The listing builds one solid part. Answer for the finished solid, in the listing's coordinates (mm). A direction names the side the tool comes from. Give positions to 0.01 mm unless a question says otherwise; leave off trailing zeros. Return JSON: item names as keys, results as strings.
from build123d import *

# Parameters (mm, degrees)
CYLINDER014005872_R                            = 40.05
CYLINDER014005872_DEPTH                        = 16
CYLINDER014005874_R                            = 3.65
CYLINDER014005874_DEPTH                        = 4
CYLINDER014005873_R                            = 2.15
CYLINDER014005873_DEPTH                        = 24
FUSION001089102007007003001_PLACEMENT_ANGLE    = 60
FUSION001089102007007003002_PLACEMENT_ANGLE    = 120
FUSION001089102007007003003_PLACEMENT_ANGLE    = 180
FUSION001089102007007003004_PLACEMENT_ANGLE    = 240
FUSION001089102007007003005_PLACEMENT_ANGLE    = 60
BOX002_W                                       = 7
BOX002_H                                       = 10
BOX002_DEPTH                                   = 3.4
PRISM003_DEPTH                                 = 3.4
CYLINDER014005875_R                            = 2.15
CYLINDER014005875_DEPTH                        = 16
FUSION001089102007007003008001_PLACEMENT_ANGLE = 60
FUSION001089102007007003008002_PLACEMENT_ANGLE = 120
FUSION001089102007007003008003_PLACEMENT_ANGLE = 180
FUSION001089102007007003008004_PLACEMENT_ANGLE = 240
FUSION001089102007007003008005_PLACEMENT_ANGLE = 60
BOX003_W                                       = 4.1
BOX003_H                                       = 8
BOX003_DEPTH                                   = 10
CYLINDER014005876_R                            = 2.65
CYLINDER014005876_DEPTH                        = 14
PRISM004_DEPTH                                 = 4.2
BOX004_W                                       = 4.1
BOX004_H                                       = 8
BOX004_DEPTH                                   = 10
CYLINDER014005877_R                            = 2.65
CYLINDER014005877_DEPTH                        = 14
PRISM005_DEPTH                                 = 4.2
CYLINDER014005871_R                            = 36
CYLINDER014005871_DEPTH                        = 16
BOX_W                                          = 10
BOX_H                                          = 44
BOX_DEPTH                                      = 16
CYLINDER014005870_R                            = 53
CYLINDER014005870_DEPTH                        = 16
CHAMFER012_SIZE                                = 0.75


with BuildPart() as obj1:
    # Cylinder014005872 → Cylinder014005872 (new body)
    with BuildSketch(Plane.XY.offset(0.1)):
        Circle(CYLINDER014005872_R)
    extrude(amount=CYLINDER014005872_DEPTH)


with BuildPart() as obj2:
    # Cylinder014005874 → Cylinder014005874 (new body)
    with BuildSketch(Plane(origin=(45, 0, 4), x_dir=(1, 0, 0), z_dir=(0, 0, 1))):
        Circle(CYLINDER014005874_R)
    extrude(amount=CYLINDER014005874_DEPTH)


with BuildPart() as obj3:
    # Cylinder014005873 → Cylinder014005873 (new body)
    with BuildSketch(Plane(origin=(45, 0, -16), x_dir=(1, 0, 0), z_dir=(0, 0, 1))):
        Circle(CYLINDER014005873_R)
    extrude(amount=CYLINDER014005873_DEPTH)

    # Fusion001089102007007003: union obj2
    add(obj2.part)


with BuildPart() as obj4:
    # Fusion001089102007007003001 base: copy of obj3
    add(obj3.part)


with BuildPart() as obj4_1:
    # Fusion001089102007007003001 placement: moved
    add(obj4.part.rotate(Axis((0, 0, 0), (0, 0, 1)), FUSION001089102007007003001_PLACEMENT_ANGLE))


with BuildPart() as obj5:
    # Fusion001089102007007003002 base: copy of obj3
    add(obj3.part)


with BuildPart() as obj5_1:
    # Fusion001089102007007003002 placement: moved
    add(obj5.part.rotate(Axis((0, 0, 0), (0, 0, 1)), FUSION001089102007007003002_PLACEMENT_ANGLE))


with BuildPart() as obj6:
    # Fusion001089102007007003003 base: copy of obj3
    add(obj3.part)


with BuildPart() as obj6_1:
    # Fusion001089102007007003003 placement: moved
    add(obj6.part.rotate(Axis((0, 0, 0), (0, 0, 1)), FUSION001089102007007003003_PLACEMENT_ANGLE))


with BuildPart() as obj7:
    # Fusion001089102007007003004 base: copy of obj3
    add(obj3.part)


with BuildPart() as obj7_1:
    # Fusion001089102007007003004 placement: moved
    add(obj7.part.rotate(Axis((0, 0, 0), (0, 0, 1)), FUSION001089102007007003004_PLACEMENT_ANGLE))


with BuildPart() as obj8:
    # Fusion001089102007007003005 base: copy of obj3
    add(obj3.part)


with BuildPart() as obj8_1:
    # Fusion001089102007007003005 placement: moved
    add(obj8.part.rotate(Axis((0, 0, 0), (0, 0, -1)), FUSION001089102007007003005_PLACEMENT_ANGLE))


with BuildPart() as fusion001089102007007003006:
    # Fusion001089102007007003006 base: copy of obj3
    add(obj3.part)

    # Fusion001089102007007003006: union obj4, obj5, obj6, obj7, obj8
    add(obj4_1.part)
    add(obj5_1.part)
    add(obj6_1.part)
    add(obj7_1.part)
    add(obj8_1.part)


with BuildPart() as krychle002:
    # Box002 → Box002 (new body)
    with BuildSketch(Plane(origin=(-3.5, 0, 0), x_dir=(1, 0, 0), z_dir=(0, 0, 1))):
        with Locations((3.5, 5)):
            Rectangle(BOX002_W, BOX002_H)
    extrude(amount=BOX002_DEPTH)


with BuildPart() as m4x003:
    # prism003 → prism003 (new body)
    with BuildSketch(Plane(origin=(0, 0, 0), x_dir=(0, 1, 0), z_dir=(0, 0, 1))):
        Polygon((4.21, 0), (2.105, 3.645967), (-2.105, 3.645967), (-4.21, 0), (-2.105, -3.645967), (2.105, -3.645967), align=None)
    extrude(amount=PRISM003_DEPTH)


with BuildPart() as m4nut:
    # Cylinder014005875 → Cylinder014005875 (new body)
    with BuildSketch(Plane.XY.offset(-8)):
        Circle(CYLINDER014005875_R)
    extrude(amount=CYLINDER014005875_DEPTH)

    # Fusion001089102007007003008: union Krychle002, M4X003
    add(krychle002.part)
    add(m4x003.part)


with BuildPart() as m4nut_1:
    # Fusion001089102007007003008 placement: moved
    add(m4nut.part.moved(Location((0, -45, 0))))


with BuildPart() as m4nut001:
    # Fusion001089102007007003008001 base: copy of M4nut
    add(m4nut_1.part)


with BuildPart() as m4nut001_1:
    # Fusion001089102007007003008001 placement: moved
    add(m4nut001.part.rotate(Axis((0, 0, 0), (0, 0, 1)), FUSION001089102007007003008001_PLACEMENT_ANGLE))


with BuildPart() as m4nut002:
    # Fusion001089102007007003008002 base: copy of M4nut
    add(m4nut_1.part)


with BuildPart() as m4nut002_1:
    # Fusion001089102007007003008002 placement: moved
    add(m4nut002.part.rotate(Axis((0, 0, 0), (0, 0, 1)), FUSION001089102007007003008002_PLACEMENT_ANGLE))


with BuildPart() as m4nut003:
    # Fusion001089102007007003008003 base: copy of M4nut
    add(m4nut_1.part)


with BuildPart() as m4nut003_1:
    # Fusion001089102007007003008003 placement: moved
    add(m4nut003.part.rotate(Axis((0, 0, 0), (0, 0, 1)), FUSION001089102007007003008003_PLACEMENT_ANGLE))


with BuildPart() as m4nut004:
    # Fusion001089102007007003008004 base: copy of M4nut
    add(m4nut_1.part)


with BuildPart() as m4nut004_1:
    # Fusion001089102007007003008004 placement: moved
    add(m4nut004.part.rotate(Axis((0, 0, 0), (0, 0, 1)), FUSION001089102007007003008004_PLACEMENT_ANGLE))


with BuildPart() as m4nut005:
    # Fusion001089102007007003008005 base: copy of M4nut
    add(m4nut_1.part)


with BuildPart() as m4nut005_1:
    # Fusion001089102007007003008005 placement: moved
    add(m4nut005.part.rotate(Axis((0, 0, 0), (0, 0, -1)), FUSION001089102007007003008005_PLACEMENT_ANGLE))


with BuildPart() as fusion001089102007007003008006:
    # Fusion001089102007007003008006 base: copy of M4nut
    add(m4nut_1.part)

    # Fusion001089102007007003008006: union M4nut001, M4nut002, M4nut003, M4nut004, M4nut005
    add(m4nut001_1.part)
    add(m4nut002_1.part)
    add(m4nut003_1.part)
    add(m4nut004_1.part)
    add(m4nut005_1.part)


with BuildPart() as krychle003:
    # Box003 → Box003 (new body)
    with BuildSketch(Plane(origin=(0, -4, 0), x_dir=(1, 0, 0), z_dir=(0, 0, 1))):
        with Locations((2.05, 4)):
            Rectangle(BOX003_W, BOX003_H)
    extrude(amount=BOX003_DEPTH)


with BuildPart() as obj9:
    # Cylinder014005876 → Cylinder014005876 (new body)
    with BuildSketch(Plane(origin=(-4, 0, 0), x_dir=(0, 0, -1), z_dir=(1, 0, 0))):
        Circle(CYLINDER014005876_R)
    extrude(amount=CYLINDER014005876_DEPTH)


with BuildPart() as m5:
    # prism004 → prism004 (new body)
    with BuildSketch(Plane(origin=(0, 0, 0), x_dir=(0, 0, -1), z_dir=(1, 0, 0))):
        Polygon((4.6, 0), (2.3, 3.983717), (-2.3, 3.983717), (-4.6, 0), (-2.3, -3.983717), (2.3, -3.983717), align=None)
    extrude(amount=PRISM004_DEPTH)

    # Fusion001089102007007003008007: union Krychle003, obj9
    add(krychle003.part)
    add(obj9.part)


with BuildPart() as m5_1:
    # Fusion001089102007007003008007 placement: moved
    add(m5.part.moved(Location((45, 15, 0))))


with BuildPart() as krychle004:
    # Box004 → Box004 (new body)
    with BuildSketch(Plane(origin=(0, -4, 0), x_dir=(1, 0, 0), z_dir=(0, 0, 1))):
        with Locations((2.05, 4)):
            Rectangle(BOX004_W, BOX004_H)
    extrude(amount=BOX004_DEPTH)


with BuildPart() as obj10:
    # Cylinder014005877 → Cylinder014005877 (new body)
    with BuildSketch(Plane(origin=(-4, 0, 0), x_dir=(0, 0, -1), z_dir=(1, 0, 0))):
        Circle(CYLINDER014005877_R)
    extrude(amount=CYLINDER014005877_DEPTH)


with BuildPart() as m006:
    # prism005 → prism005 (new body)
    with BuildSketch(Plane(origin=(0, 0, 0), x_dir=(0, 0, -1), z_dir=(1, 0, 0))):
        Polygon((4.6, 0), (2.3, 3.983717), (-2.3, 3.983717), (-4.6, 0), (-2.3, -3.983717), (2.3, -3.983717), align=None)
    extrude(amount=PRISM005_DEPTH)

    # Fusion001089102007007003008008: union Krychle004, obj10
    add(krychle004.part)
    add(obj10.part)


with BuildPart() as m006_1:
    # Fusion001089102007007003008008 placement: moved
    add(m006.part.moved(Location((45, -15, 0))))


with BuildPart() as fusion001089102007007002:
    # Cylinder014005871 → Cylinder014005871 (new body)
    with BuildSketch(Plane.XY.offset(-8)):
        Circle(CYLINDER014005871_R)
    extrude(amount=CYLINDER014005871_DEPTH)

    # Fusion001089102007007002: union obj1, Fusion001089102007007003006, Fusion001089102007007003008006, M5, M006
    add(obj1.part)
    add(fusion001089102007007003006.part)
    add(fusion001089102007007003008006.part)
    add(m5_1.part)
    add(m006_1.part)


with BuildPart() as krychle:
    # Box → Box (new body)
    with BuildSketch(Plane(origin=(43, -22, -8), x_dir=(1, 0, 0), z_dir=(0, 0, 1))):
        with Locations((5, 22)):
            Rectangle(BOX_W, BOX_H)
    extrude(amount=BOX_DEPTH)


with BuildPart() as obj11:
    # Cylinder014005870 → Cylinder014005870 (new body)
    with BuildSketch(Plane.XY.offset(-8)):
        Circle(CYLINDER014005870_R)
    extrude(amount=CYLINDER014005870_DEPTH)

    # Fusion001089102007007003007: union Krychle
    add(krychle.part)

    # Cut009003003009003: cut Fusion001089102007007002
    add(fusion001089102007007002.part, mode=Mode.SUBTRACT)

    # Chamfer012
    chamfer012_edges = [obj11.edges().sort_by_distance(p)[0] for p in [
        (-53, 0, 8),
        (-53, 0, -8),
        (50.609127, 22, -8),
        (50.609127, 22, 8),
        (50.609127, -22, -8),
        (50.609127, -22, 8),
        (53, 0, -8),
        (-36, 0, -8),
        (-40.05, 0, 8),
        (53, 0, 8),
    ]]
    chamfer(chamfer012_edges, length=CHAMFER012_SIZE)


solid = obj11.part
Item 1: Given pin 1 Ø4 at (x, z) = (51, -1.5) entering from -Y; pin 2 Ø4 at (x, z) = (-15.5, 3) entering from -Y; pin 3 Ø1.7 at (y, z) = (-44.5, 2.5) entering from +X, each flat-ended and moving along its own axis, determine where each tip first touches the part or whether it passes through.
Geometry results:
{"pin 1": "stops at y = -22", "pin 2": "stops at y = -51.25", "pin 3": "stops at x = 30.06"}
Item 2: Determine the mould class of faces 1 (the flat face through (47, -11.016, -1)), 2 (the flat face through (-16, -38, 8)) for opening direction Y: +Y half, -Y half, draft (parallel to the pull), parting line (faces both ways), or undercut.
Geometry results:
{"face 1": "undercut", "face 2": "draft"}
Item 3: Find the intervals of material crossed by line 1 (Y direction, x = 0, z = 3.5); line 2 (X direction, y = 0.5, z = -2); line 3 (Z direction, x = 50, y = -15), in increasing order.
Geometry results:
{"line 1": "y = -53 to -47.15, -42.85 to -40.05, 40.05 to 42.85, 47.15 to 53", "line 2": "x = -53 to -47.09, -42.91 to -36, 36 to 42.91, 47.09 to 53", "line 3": "z = -8 to -2.65, 2.65 to 8"}
Item 4: Which of the six approach directions +Z, -Z, +X, -X, +Y, -Y give full straight-line access (tool end or side, diameter ignored) to faces 3 (the flat face through (-1.8, 48.17, 1.68)), 4 (the cylindrical face through (22.78, 36.84, -2.08)), 5 (the flat face through (45, -15, 3))?
Geometry results:
{"face 3": "none", "face 4": "+Z, -Z", "face 5": "+Z"}
